```python
from build123d import *

# Parameters (mm, degrees)
F0_W     = 27
F0_H     = 27
F1_DEPTH = 500
F3_DEPTH = 27.001
F4_DEPTH = 27.001
F5_SIZE  = 2
F6_R     = 2


with BuildPart() as f1:
    # F0 (on Front) → F1 (new body, symmetric)
    with BuildSketch(Plane.XZ):
        with Locations((13.5, 13.5)):
            Rectangle(F0_W, F0_H)
    extrude(amount=F1_DEPTH, both=True)

    # F2 (on face) → F3 (cut, through all)
    with BuildSketch(Plane.XY.offset(27)):
        with BuildLine():
            Line((18.5, -500), (18.5, -488))
            ThreePointArc((18.5, -488), (13.5, -483), (8.5, -488))
            Line((8.5, -488), (8.5, -500))
            Line((8.5, -500), (18.5, -500))
        make_face()
    extrude(amount=-F3_DEPTH, mode=Mode.SUBTRACT)

    # F2 (on face) → F4 (cut, through all)
    with BuildSketch(Plane.XY.offset(27)):
        with BuildLine():
            Line((18.5, -500), (18.5, -488))
            ThreePointArc((18.5, -488), (13.5, -483), (8.5, -488))
            Line((8.5, -488), (8.5, -500))
            Line((8.5, -500), (18.5, -500))
        make_face()
        with BuildLine():
            ThreePointArc((8.5, 488), (13.5, 483), (18.5, 488))
            Line((18.5, 488), (18.5, 500))
            Line((18.5, 500), (8.5, 500))
            Line((8.5, 500), (8.5, 488))
        make_face()
    extrude(amount=-F4_DEPTH, mode=Mode.SUBTRACT)

    # F5
    f5_edges = [f1.edges().sort_by_distance(p)[0] for p in [
        (0, -500, 13.5),
        (27, -500, 13.5),
        (0, 500, 13.5),
        (27, 500, 13.5),
    ]]
    chamfer(f5_edges, length=F5_SIZE)

    # F6
    f6_edges = [f1.edges().sort_by_distance(p)[0] for p in [
        (21.75, -500, 27),
        (26, -499, 27),
        (18.5, -494, 27),
        (27, 0, 27),
        (13.5, -483, 27),
        (26, 499, 27),
        (8.5, -494, 27),
        (21.75, 500, 27),
        (5.25, -500, 27),
        (18.5, 494, 27),
        (1, -499, 27),
        (13.5, 483, 27),
        (0, 0, 27),
        (8.5, 494, 27),
        (1, 499, 27),
        (5.25, 500, 27),
        (0, 0, 0),
        (1, 499, 0),
        (1, -499, 0),
        (5.25, 500, 0),
        (5.25, -500, 0),
        (8.5, 494, 0),
        (8.5, -494, 0),
        (13.5, 483, 0),
        (13.5, -483, 0),
        (18.5, 494, 0),
        (18.5, -494, 0),
        (21.75, 500, 0),
        (21.75, -500, 0),
        (26, 499, 0),
        (26, -499, 0),
        (27, 0, 0),
        (18.5, 500, 13.5),
        (8.5, 500, 13.5),
        (18.5, -500, 13.5),
        (8.5, -500, 13.5),
    ]]
    fillet(f6_edges, radius=F6_R)


solid = f1.part
```
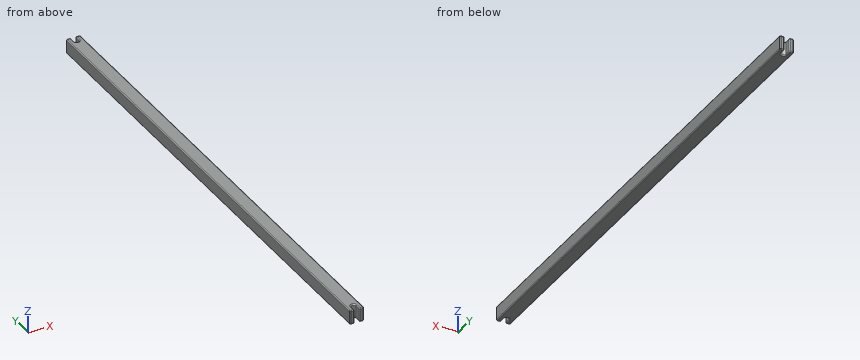
Read the model definition and answer for the solid it produces. Units are mm, in the model's axes. Give positions to 0.01 mm unless a question says otherwise; leave off trailing zeros. Loops run counter-clockwise (first coordinate to the right, second up) from the corner with the lowest first, then second, coordinate; pieces in that order, holes last.
Item 1: The part is cut by section A-A (x = 13.5). Write down the section's boundary in (y, z), and give its area (3 significant figures).
Item 2: Find the intervals of material crossed by line 1 along Y through (x, z) = (13.5, 19); line 2 along Y through (x, z) = (14.25, 16.5), in increasing order.
Item 3: This flat-tipped pin is pushed along its axis until it touches: pin 1 Ø4 at (x, y) = (12.5, 263) entering from -Z. Where does it stop, or does it pass through?
Taken from the geometry:
1. outline: (-483, 2) arc R2 ccw to (-481, 0) - (481, 0) arc R2 ccw to (483, 2) - (483, 25) arc R2 ccw to (481, 27) - (-481, 27) arc R2 ccw to (-483, 25) - close
1. area: 26,100 mm2
2. line 1: y = -483 to 483
2. line 2: y = -483.06 to 483.06
3. pin 1: stops at z = 0
